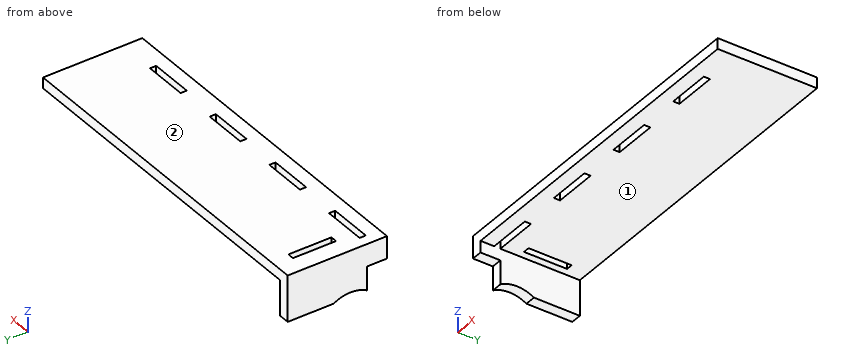
Autodesk Inventor part; units mm, degrees
ref_plane "YZ Plane" through (0, 0, 0) normal (1, 0, 0) x (0, 1, 0)
ref_plane "XZ Plane" through (0, 0, 0) normal (0, 1, 0) x (-1, 0, 0)
ref_plane "XY Plane" through (0, 0, 0) normal (0, 0, 1) x (1, 0, 0)
sketch "Sketch1" plane through (0, 0, 0) normal (0, 0, 1) x (1, 0, 0)
  line L0 (-96.8016, -0.4814) -> (101.2834, -0.4814)
  line L1 (101.2834, -0.4814) -> (101.2834, -56.7314)
  line L2 (101.2834, -56.7314) -> (-96.8016, -56.7314)
  line L3 (-96.8016, -56.7314) -> (-96.8016, -0.4814)
  line L4 (-96.8016, -0.4814) -> (-90.7166, -0.4814)
  line L5 (-90.7166, -0.4814) -> (-90.7166, -56.7314)
  line L6 (-90.7166, -56.7314) -> (-96.8016, -56.7314)
  line L7 (-96.8016, -56.7314) -> (-96.8016, -0.4814)
  line L8 (-86.5466, -10.6314) -> (-82.8466, -10.6314)
  line L9 (-82.8466, -10.6314) -> (-82.8466, -35.0314)
  line L10 (-82.8466, -35.0314) -> (-86.5466, -35.0314)
  line L11 (-86.5466, -35.0314) -> (-86.5466, -10.6314)
  line L12 (-90.7166, -45.4814) -> (-65.9666, -45.4814)
  line L13 (-65.9666, -45.4814) -> (-65.9666, -48.9814)
  line L14 (-65.9666, -48.9814) -> (-90.7166, -48.9814)
  line L15 (-90.7166, -48.9814) -> (-90.7166, -45.4814)
  line L16 (-17.6566, -45.4814) -> (-17.6566, -48.9814)
  line L17 (-17.6566, -48.9814) -> (-42.4066, -48.9814)
  line L18 (-42.4066, -48.9814) -> (-42.4066, -45.4814)
  line L19 (-42.4066, -45.4814) -> (-17.6566, -45.4814)
  line L20 (30.6534, -45.4814) -> (30.6534, -48.9814)
  line L21 (30.6534, -48.9814) -> (5.9034, -48.9814)
  line L22 (5.9034, -48.9814) -> (5.9034, -45.4814)
  line L23 (5.9034, -45.4814) -> (30.6534, -45.4814)
  line L24 (78.9634, -45.4814) -> (78.9634, -48.9814)
  line L25 (78.9634, -48.9814) -> (54.2134, -48.9814)
  line L26 (54.2134, -48.9814) -> (54.2134, -45.4814)
  line L27 (54.2134, -45.4814) -> (78.9634, -45.4814)
  point P0 (0, 0)
  dimension "d0" = 198.085
  dimension "d1" = 56.25
  dimension "d2" = 0
  dimension "d3" = 0
  dimension "d4" = 0
  dimension "d5" = 6.085
  dimension "d6" = 4.17
  dimension "d7" = 10.15
  dimension "d8" = 3.7
  dimension "d9" = 24.4
  dimension "d10" = 7.75
  dimension "d11" = 0
  dimension "d12" = 24.75
  dimension "d15" = 48.31
  dimension "d20" = 3.5
extrude "Extrusion1" add sketch "Sketch1" against normal blind 6.085 contours L0 L1 L2 L5 L14 L13 L12
extrude "Extrusion2" add sketch "Sketch1" against normal blind 26.125 contours L0 L5 L2 L3
sketch "Sketch2" plane through (-96.8016, -56.7314, 0) normal (-1, 0, 0) x (0, 0, 1)
  line L0 (0, 0) -> (-84, 0)
  circle A0 centre (-42, 20.75) radius 18.5
  point P0 (0, 56.7314)
  dimension "d25" = 84
  dimension "d26" = 37
  dimension "d27" = 20.75
extrude "Extrusion3" cut sketch "Sketch2" against normal blind 26.125
sketch "Sketch3" plane through (-96.8016, -56.7314, 0) normal (-1, 0, 0) x (0, 0, 1)
  line L0 (-68.8984, 11.25) -> (-12.625, 11.25)
  line L1 (-12.625, 11.25) -> (-12.625, -13.0392)
  line L2 (-12.625, -13.0392) -> (-68.8984, -13.0392)
  line L3 (-68.8984, -13.0392) -> (-68.8984, 11.25)
  line L4 (-26.125, 0) -> (-26.125, 11.2508)
  line L5 (0, 0) -> (-26.125, 0)
  point P0 (0, 56.7314)
  dimension "d30" = 13.5
  dimension "d31" = 11.25
extrude "Extrusion4" cut sketch "Sketch3" against normal blind 10
properties part number "side frame left"
The model under review builds one solid part; all positions refer to its coordinate system, in mm. Face numbers are marked on the shaded views. A direction names the side the tool comes from. Round coordinates to 2 decimals unless told otherwise and drop trailing zeros. Write each loop counter-clockwise with the first axis right and the second up, starting at its lowest first coordinate (ties: lowest second). Pieces come first, ordered by that corner, then holes. Notation, with made-up numbers: M 46.25,68.25 L 93.25,68.25 A24 ccw 93.25,99.25 Z; hole C 40.5,5 d9. An arc over 180 degrees is marked long. Answer as CSV lines item,"result". Start each with the question number.
Q1. Wall thickness on line 1 along Y through (x, z) = (-18, -4.75); line 2 along Z through (x, y) = (66.5, -43.5) (3 decimals); line 3 along X through (y, z) = (-6.5, -11.5): over which ranges is each line inside the solid? List them lowest first.
Q2. Consider section D-D, the plane y = -7. Give the boundary of the cut face in (x, z) (3 decimals), then the cut area to 3 significant figures.
Q3. Consider section C-C, the plane y = -16.5. Give the boundary of the cut face in (x, z) (3 decimals).
Q4. Consider section A-A, the plane x = 13. Give the boundary of the cut face in (y, z) (3 decimals).
Q5. Consider section B-B, the plane z = -1.75. Give the boundary of the cut face in (x, y).
Q6. Tool access review of the marked faces 1 and 2: name each direction out of +Z, -Z, +X, -X, +Y, -Y from which nothing blocks a thin tool from reaching the whole face with its end or side.
Q7. Clearance check with flat-ended pins moving along their axes: P1, Ø5, axis at x = -74.5, y = -26.5, coming from the +Z side; P2, Ø2, axis at x = -72, y = -25.5, coming from the -Z side (3 decimals); P3, Ø3, axis at x = -68, z = -9.5, coming from the +Y side; P4, Ø3, axis at y = -7, z = -20, coming from the +X side. State where each tip first meets the part, or that it passes through.
Result set:
1,line 1,"y = -56.73 to -48.98, -45.48 to -0.48"
1,line 2,"z = -6.085 to 0"
1,line 3,"x = -96.8 to -90.72"
2,outline,"M -96.802,-26.125 L -90.717,-26.125 L -90.717,-6.085 L 101.283,-6.085 L 101.283,0 L -96.802,0 Z"
2,area,"1,330 mm²"
3,outline,"M -96.802,-26.125 L -90.717,-26.125 L -90.717,-6.085 L -86.547,-6.085 L -86.547,0 L -96.802,0 Z; M -82.847,-6.085 L 101.283,-6.085 L 101.283,0 L -82.847,0 Z"
4,outline,"M -56.731,-6.085 L -48.981,-6.085 L -48.981,0 L -56.731,0 Z; M -45.481,-6.085 L -0.481,-6.085 L -0.481,0 L -45.481,0 Z"
5,outline,"M -96.8,-56.73 L 101.28,-56.73 L 101.28,-0.48 L -96.8,-0.48 Z; hole M -90.72,-48.98 L -65.97,-48.98 L -65.97,-45.48 L -90.72,-45.48 Z; hole M -86.55,-35.03 L -82.85,-35.03 L -82.85,-10.63 L -86.55,-10.63 Z; hole M -42.41,-48.98 L -17.66,-48.98 L -17.66,-45.48 L -42.41,-45.48 Z; hole M 5.9,-48.98 L 30.65,-48.98 L 30.65,-45.48 L 5.9,-45.48 Z; hole M 54.21,-48.98 L 78.96,-48.98 L 78.96,-45.48 L 54.21,-45.48 Z"
6,face 1,"-Z, +X, +Y, -Y"
6,face 2,"+Z, +X, -X, +Y, -Y"
7,P1,"stops at z = 0"
7,P2,"stops at z = -6.085"
7,P3,"passes through"
7,P4,"stops at x = -90.72"
